Check sheet for the modelled part. Datum: model origin and axes. Units: mm. A direction names the side the tool comes from. Coordinates: 2 decimals unless noted, no trailing zeros. Loops run counter-clockwise (first coordinate to the right, second up) from the corner with the lowest first, then second, coordinate; pieces in that order, holes last.
from build123d import *

# Parameters (mm, degrees)
BOSS_EXTRU_1_DEPTH             = 2
ESQUISSE2_W                    = 16.5
ESQUISSE2_H                    = 1
ENL_V_MAT_EXTRU_1_DEPTH        = 0.75
ESQUISSE3_W                    = 16.5
ESQUISSE3_H                    = 1
ENL_V_MAT_EXTRU_2_DEPTH        = 0.75
R_P_TITION_CIRCULAIRE1_DEPTH   = 2
R_P_TITION_START               = 1
R_P_TITION_CIRCULAIRE1_2_DEPTH = 1
BOSS_EXTRU_2_DEPTH             = 1
BOSS_EXTRU_3_DEPTH             = 1


# Read off the part's stored shape, not the designer's step: Répétition circulaire1
with BuildPart() as part:
    # Esquisse1 → Boss.-Extru.1 (new body)
    with BuildSketch(Plane.XY):
        with BuildLine():
            Line((11.258330249, 6.5), (28.145825623, 16.25))
            ThreePointArc((28.145825623, 16.25), (31.392589354, 8.411618966), (32.5, 0))
            Line((32.5, 0), (13, 0))
            ThreePointArc((13, 0), (12.557035742, 3.364647586), (11.258330249, 6.5))
        make_face()
        with BuildLine():
            Line((12.915559198, 6.590776176), (27.213929282, 14.845943993))
            ThreePointArc((27.213929282, 14.845943993), (29.943700615, 8.023390398), (30.990926091, 0.75))
            Line((30.990926091, 0.75), (14.480590458, 0.75))
            ThreePointArc((14.480590458, 0.75), (14.005924481, 3.752876154), (12.915559198, 6.590776176))
        make_face(mode=Mode.SUBTRACT)
    extrude(amount=BOSS_EXTRU_1_DEPTH)

    # Esquisse2 → Enlèv. mat.-Extru.1 (cut)
    with BuildSketch(Plane(origin=(0, 0, 0), x_dir=(0.866025403784438, 0.5000000000000011, 0), z_dir=(-0.5000000000000011, 0.8660254037844382, 0))):
        with Locations((22.75, -0.5)):
            Rectangle(ESQUISSE2_W, ESQUISSE2_H)
    extrude(amount=-ENL_V_MAT_EXTRU_1_DEPTH, mode=Mode.SUBTRACT)

    # Esquisse3 → Enlèv. mat.-Extru.2 (cut)
    with BuildSketch(Plane.XZ):
        with Locations((22.75, 0.5)):
            Rectangle(ESQUISSE3_W, ESQUISSE3_H)
    extrude(amount=-ENL_V_MAT_EXTRU_2_DEPTH, mode=Mode.SUBTRACT)

    # Répétition circulaire1 outline → Répétition circulaire1 (add)
    with BuildSketch(Plane.XY):
        with BuildLine():
            Line((14.500000002, 0), (13, 0))
            ThreePointArc((13, 0), (-3.363880515, -12.557241253), (-11.25912429, 6.498624487))
            Line((-11.25912429, 6.498624487), (-12.558254016, 7.248465774))
            Line((-12.558254016, 7.248465774), (-12.933174659, 6.598900911))
            Line((-12.933174659, 6.598900911), (-12.916364317, 6.589198194))
            ThreePointArc((-12.916364317, 6.589198194), (-14.006382877, 3.75116498), (-14.480681979, 0.748230857))
            Line((-14.480681979, 0.748230857), (-14.500091522, 0.748228486))
            Line((-14.500091522, 0.748228486), (-14.499999892, -0.001771509))
            Line((-14.499999892, -0.001771509), (-14.499921381, -0.751518432))
            Line((-14.499921381, -0.751518432), (-14.480511838, -0.7515164))
            ThreePointArc((-14.480511838, -0.7515164), (-14.005531404, -3.75434283), (-12.914868943, -6.592128654))
            Line((-12.914868943, -6.592128654), (-12.931677083, -6.601835185))
            Line((-12.931677083, -6.601835185), (-12.556609068, -7.251314965))
            Line((-12.556609068, -7.251314965), (-12.181678945, -7.900582135))
            Line((-12.181678945, -7.900582135), (-12.164870636, -7.890875897))
            ThreePointArc((-12.164870636, -7.890875897), (-10.252153541, -10.253943035), (-7.888752606, -12.166247668))
            Line((-7.888752606, -12.166247668), (-7.898455911, -12.183057672))
            Line((-7.898455911, -12.183057672), (-7.248904135, -12.558000989))
            Line((-7.248904135, -12.558000989), (-6.599578081, -12.932829124))
            Line((-6.599578081, -12.932829124), (-6.589874484, -12.91601929))
            ThreePointArc((-6.589874484, -12.91601929), (-3.751898347, -14.006186447), (-0.748989062, -14.480642782))
            Line((-0.748989062, -14.480642782), (-0.748987707, -14.500052325))
            Line((-0.748987707, -14.500052325), (0.001012291, -14.499999965))
            Line((0.001012291, -14.499999965), (0.750759217, -14.49996071))
            Line((0.750759217, -14.49996071), (0.750758201, -14.480551168))
            ThreePointArc((0.750758201, -14.480551168), (3.753609497, -14.005727962), (6.591452424, -12.915214088))
            Line((6.591452424, -12.915214088), (6.601158075, -12.932022737))
            Line((6.601158075, -12.932022737), (7.250657492, -12.556988728))
            Line((7.250657492, -12.556988728), (7.899944293, -12.182092602))
            Line((7.899944293, -12.182092602), (7.890238935, -12.165283784))
            ThreePointArc((7.890238935, -12.165283784), (10.25340622, -10.252690422), (12.165834597, -7.889389619))
            Line((12.165834597, -7.889389619), (12.182644093, -7.899093804))
            Line((12.182644093, -7.899093804), (12.55762142, -7.249561661))
            Line((12.55762142, -7.249561661), (12.932483553, -6.600255234))
            Line((12.932483553, -6.600255234), (12.915674227, -6.590550756))
            ThreePointArc((12.915674227, -6.590550756), (14.005989979, -3.752631704), (14.480603545, -0.749747266))
            Line((14.480603545, -0.749747266), (14.500013088, -0.749746927))
            Line((14.500013088, -0.749746927), (14.500000002, 0))
        make_face()
        with BuildLine():
            Line((32.5, 0), (31.000000004, 0))
            Line((31.000000004, 0), (31.000013085, -0.749458948))
            Line((31.000013085, -0.749458948), (30.990939177, -0.749459106))
            ThreePointArc((30.990939177, -0.749459106), (29.943840645, -8.022867781), (27.214188388, -14.845469018))
            Line((27.214188388, -14.845469018), (27.222046703, -14.850005835))
            Line((27.222046703, -14.850005835), (26.847328557, -15.499062863))
            Line((26.847328557, -15.499062863), (26.472351226, -16.148595003))
            Line((26.472351226, -16.148595003), (26.464492832, -16.144058323))
            ThreePointArc((26.464492832, -16.144058323), (21.921075367, -21.91954504), (16.145905854, -26.4633657))
            Line((16.145905854, -26.4633657), (16.150443083, -26.471223777))
            Line((16.150443083, -26.471223777), (15.501405676, -26.845975906))
            Line((15.501405676, -26.845975906), (14.851906256, -27.221009911))
            Line((14.851906256, -27.221009911), (14.847368891, -27.213151913))
            ThreePointArc((14.847368891, -27.213151913), (8.024958236, -29.94328047), (0.75162268, -30.990886779))
            Line((0.75162268, -30.990886779), (0.751623155, -30.999960688))
            Line((0.751623155, -30.999960688), (0.002164208, -30.999999929))
            Line((0.002164208, -30.999999929), (-0.74783579, -31.000052284))
            Line((-0.74783579, -31.000052284), (-0.747836423, -30.990978376))
            ThreePointArc((-0.747836423, -30.990978376), (-8.021299914, -29.94426068), (-14.844044066, -27.214965658))
            Line((-14.844044066, -27.214965658), (-14.848580472, -27.22282421))
            Line((-14.848580472, -27.22282421), (-15.497657119, -26.848140049))
            Line((-15.497657119, -26.848140049), (-16.147208892, -26.473196728))
            Line((-16.147208892, -26.473196728), (-16.142672624, -26.465338097))
            ThreePointArc((-16.142672624, -26.465338097), (-21.918397225, -21.922223041), (-26.462520266, -16.147291451))
            Line((-26.462520266, -16.147291451), (-26.470378105, -16.151829091))
            Line((-26.470378105, -16.151829091), (-26.845164218, -15.502811306))
            Line((-26.845164218, -15.502811306), (-27.220232229, -14.853331525))
            Line((-27.220232229, -14.853331525), (-27.212374469, -14.848793747))
            ThreePointArc((-27.212374469, -14.848793747), (-29.942860243, -8.026526051), (-30.990847382, -0.753245358))
            Line((-30.990847382, -0.753245358), (-30.99992129, -0.753246308))
            Line((-30.99992129, -0.753246308), (-30.999999773, -0.003787364))
            Line((-30.999999773, -0.003787364), (-31.000091398, 0.74621263))
            Line((-31.000091398, 0.74621263), (-30.99101749, 0.746213739))
            ThreePointArc((-30.99101749, 0.746213739), (-29.944680634, 8.019732025), (-27.215742853, 14.842619073))
            Line((-27.215742853, 14.842619073), (-27.223601643, 14.847155068))
            Line((-27.223601643, 14.847155068), (-26.848680999, 15.49671993))
            Line((-26.848680999, 15.49671993), (-28.147810725, 16.246561217))
            ThreePointArc((-28.147810725, 16.246561217), (-8.409701286, -31.393103132), (32.5, 0))
        make_face()
    extrude(amount=R_P_TITION_CIRCULAIRE1_DEPTH)

    # R_p_tition circulaire1 2 outline → R_p_tition circulaire1 2 (add)
    with BuildSketch(Plane.XY.offset(R_P_TITION_START)):
        Polygon((31.000000004, 0), (14.500000002, 0), (14.500013088, -0.749746927), (30.990939177, -0.749459106), (31.000013085, -0.749458948), align=None)
        Polygon((-12.933174659, 6.598900911), (-12.558254016, 7.248465774), (-26.848680999, 15.49671993), (-27.223601643, 14.847155068), (-27.215742853, 14.842619073), align=None)
        Polygon((27.222046703, -14.850005835), (27.214188388, -14.845469018), (12.932483553, -6.600255234), (12.557621422, -7.249561662), (12.182644093, -7.899093803), (26.464492832, -16.144058323), (26.472351226, -16.148595003), (26.847328553, -15.499062861), align=None)
        Polygon((-14.500091522, 0.748228486), (-30.99101749, 0.746213739), (-31.000091398, 0.74621263), (-30.999999769, -0.003787364), (-30.99992129, -0.753246308), (-30.990847382, -0.753245358), (-14.499921381, -0.751518433), (-14.499999894, -0.001771509), align=None)
        Polygon((16.150443083, -26.471223777), (16.145905854, -26.4633657), (7.899944293, -12.182092602), (7.250657493, -12.55698873), (6.601158075, -12.932022737), (14.84736889, -27.213151913), (14.851906256, -27.221009911), (15.501405673, -26.845975902), align=None)
        Polygon((-12.931677083, -6.601835185), (-27.212374469, -14.848793747), (-27.220232229, -14.853331525), (-26.845164214, -15.502811304), (-26.470378105, -16.151829091), (-26.462520266, -16.147291451), (-12.181678945, -7.900582135), (-12.55660907, -7.251314966), align=None)
        Polygon((0.751623155, -30.999960688), (0.75162268, -30.990886779), (0.750759217, -14.49996071), (0.001012291, -14.499999967), (-0.748987707, -14.500052325), (-0.747836423, -30.990978376), (-0.74783579, -31.000052284), (0.002164208, -30.999999924), align=None)
        Polygon((-7.898455911, -12.183057672), (-16.142672624, -26.465338097), (-16.147208892, -26.473196728), (-15.497657117, -26.848140045), (-14.848580472, -27.22282421), (-14.844044066, -27.214965658), (-6.599578081, -12.932829124), (-7.248904136, -12.558000991), align=None)
    extrude(amount=R_P_TITION_CIRCULAIRE1_2_DEPTH)

    # Esquisse5 → Boss.-Extru.2 (add)
    with BuildSketch(Plane(origin=(0, 0, 0), x_dir=(0.866025403784438, 0.5000000000000011, 0), z_dir=(-0.5000000000000011, 0.8660254037844382, 0))):
        Polygon((32.5, 0), (31, 0), (31, -1), (14.5, -1), (14.5, 0), (13, 0), (13, -2), (32.5, -2), align=None)
    extrude(amount=BOSS_EXTRU_2_DEPTH)

    # Esquisse6 → Boss.-Extru.3 (add)
    with BuildSketch(Plane(origin=(0, 0, 0), x_dir=(0.8660864838448452, -0.4998941913057929, 0), z_dir=(0.49989419130579293, 0.8660864838448453, 0))):
        Polygon((-14.5, -1), (-31, -1), (-31, 0), (-32.5, 0), (-32.5, -2), (-13, -2), (-13, 0), (-14.5, 0), align=None)
    extrude(amount=BOSS_EXTRU_3_DEPTH)


solid = part.part
(1) Section check A-A, the plane x = -22. Enter the section's corners in (y, z), plus the area to 3 significant figures.
(2) Draft check along X on faces 1 (the face through (-7.92, -29.97, 0.99)), 2 (the face through (-1.3, -13.1, 0)). Enter one of: pulls with the +X half, pulls with the -X half, needs draft (parallel to the pull), parting line crosses it, or undercut.
(3) Gauge pin test, flat ends, axial feed: P1, Ø0.8, axis at y = -21, z = 1.5, coming from the +X side; P2, Ø5, axis at x = -16, y = -11, coming from the -Z side; P3, Ø0.8, axis at x = 26.5, z = 1.5, coming from the -Y side. Record the tip position at first contact, or that the pin passes through.
(4) Section check B-B, the plane y = -25. Enter the section's corners in (x, z).
(5) Section check C-C, the plane y = 14. Enter the section's corners in (x, z).
(6) Scan lines: line 1 along X through (y, z) = (-9, 0.85); line 2 along Y through (x, z) = (19, 1.8); line 3 along X through (y, z) = (12.5, 1.65). Record each from-to range of solid material in increasing order.
(7) Set-up check for faces 3 (the face through (-19.322, 12.307, 1.43)), 4 (the face through (11, -20, 1)), 5 (the face through (19.96, 10.66, 1.65)): record each of +Z, -Z, +X, -X, +Y, -Y from which the full face is reachable in a straight line by a thin tool's end or side.
Determined:
1. outline: (-23.92, 0) - (-21.84, 0) - (-21.84, 2) - (-23.92, 2) - close; (-13.57, 1) - (-11.84, 1) - (-11.84, 2) - (-13.57, 2) - close; (-0.75, 1) - (0.75, 1) - (0.75, 2) - (-0.75, 2) - close; (11.83, 1) - (13.85, 1) - (13.85, 2) - (11.83, 2) - close
1. area: 9.41 mm2
2. face 1: undercut
2. face 2: needs draft
3. P1: stops at x = 25.14
3. P2: stops at z = 1
3. P3: stops at y = -19.37
4. outline: (-20.77, 0) - (-18.33, 0) - (-18.33, 2) - (-20.77, 2) - close; (-15.3, 1) - (-13.57, 1) - (-13.57, 2) - (-15.3, 2) - close; (-0.75, 1) - (0.75, 1) - (0.75, 2) - (-0.75, 2) - close; (13.57, 1) - (15.3, 1) - (15.3, 2) - (13.57, 2) - close; (18.33, 0) - (20.77, 0) - (20.77, 2) - (18.33, 2) - close
5. outline: (-29.33, 0) - (-27.66, 0) - (-27.66, 2) - (-29.33, 2) - close; (-25.76, 1) - (-22.26, 1) - (-22.26, 2) - (-25.76, 2) - close; (22.25, 1) - (25.75, 1) - (25.75, 2) - (22.25, 2) - close; (27.66, 0) - (29.33, 0) - (29.33, 2) - (27.66, 2) - close
6. line 1: x = -31.23 to -29.66, -11.37 to -9.38, 9.38 to 11.37, 29.66 to 31.23
6. line 2: y = -26.37 to -24.49, -11.83 to -10.1, -0.75 to 0.75, 10.1 to 12.12
6. line 3: x = -30 to -28.37, -23.16 to -19.66, 19.65 to 23.15, 28.37 to 30
7. face 3: +Z, -Z, +Y
7. face 4: -Z
7. face 5: +Z, -Z
